Source: CAD feature listing. Evaluate the final solid. Frame: model axes, mm. Face numbers are marked on the shaded views. A direction names the side the tool comes from. Give positions to 0.01 mm unless a question says otherwise; leave off trailing zeros.
from build123d import *

# Parameters (mm, degrees)
SKETCH1_R           = 21
SKETCH1_R_2         = 12
BOSS_EXTRUDE1_DEPTH = 45
SKETCH4_RX          = 60
SKETCH4_RY          = 36
SKETCH4_R           = 6
SKETCH4_R_2         = 12
BOSS_EXTRUDE2_DEPTH = 15
SKETCH5_R           = 25
BOSS_EXTRUDE3_DEPTH = 9


with BuildPart() as part:
    # Sketch1 → Boss-Extrude1 (new body)
    with BuildSketch(Plane(origin=(0, 0, 0), x_dir=(1, 0, 0), z_dir=(0, 1, 0))):
        with Locations(Location((0, 0, 0), (0, 0, 90))):
            Circle(SKETCH1_R)
        with Locations(Location((0, 0, 0), (0, 0, 90))):
            Circle(SKETCH1_R_2, mode=Mode.SUBTRACT)
    extrude(amount=BOSS_EXTRUDE1_DEPTH)

    # Sketch4 → Boss-Extrude2 (add)
    with BuildSketch(Plane(origin=(0, 45, 0), x_dir=(1, 0, 0), z_dir=(0, 1, 0))):
        with Locations((0, 0)):
            Ellipse(SKETCH4_RX, SKETCH4_RY)
        with Locations(Location((-42, 0, 0), (0, 0, 270))):
            Circle(SKETCH4_R, mode=Mode.SUBTRACT)
        with Locations(Location((42, 0, 0), (0, 0, 90))):
            Circle(SKETCH4_R, mode=Mode.SUBTRACT)
        with Locations(Location((0, 0, 0), (0, 0, 90))):
            Circle(SKETCH4_R_2, mode=Mode.SUBTRACT)
    extrude(amount=BOSS_EXTRUDE2_DEPTH)

    # Sketch5 → Boss-Extrude3 (add)
    with BuildSketch(Plane(origin=(0, 60, 0), x_dir=(1, 0, 0), z_dir=(0, 1, 0))):
        with Locations(Location((0, 0, 0), (0, 0, 270))):
            Circle(SKETCH5_R)
    extrude(amount=BOSS_EXTRUDE3_DEPTH)

    # Sketch6 → Cut-Revolve1 (revolve, cut)
    with BuildSketch(Plane.XY, mode=Mode.PRIVATE) as cut_revolve1_sk:
        with BuildLine():
            Line((-11.5, 57.5), (0, 57.5))
            Line((0, 57.5), (0, 80.5))
            Line((0, 80.5), (-11.5, 80.5))
            ThreePointArc((-11.5, 80.5), (-23, 69), (-11.5, 57.5))
        make_face()
    revolve(cut_revolve1_sk.sketch.rotate(Axis((0, 0, 0), (0, 1, 0)), 270), axis=Axis((0, 0, 0), (0, 1, 0)), mode=Mode.SUBTRACT)

    # Sketch7 → Cut-Revolve2 (revolve, cut)
    with BuildSketch(Plane.XY, mode=Mode.PRIVATE) as cut_revolve2_sk:
        Polygon((0, 0), (-21, 0), (0, 5.626933041), align=None)
    revolve(cut_revolve2_sk.sketch.rotate(Axis((0, 0, 0), (0, 1, 0)), 270), axis=Axis((0, 0, 0), (0, 1, 0)), mode=Mode.SUBTRACT)


solid = part.part
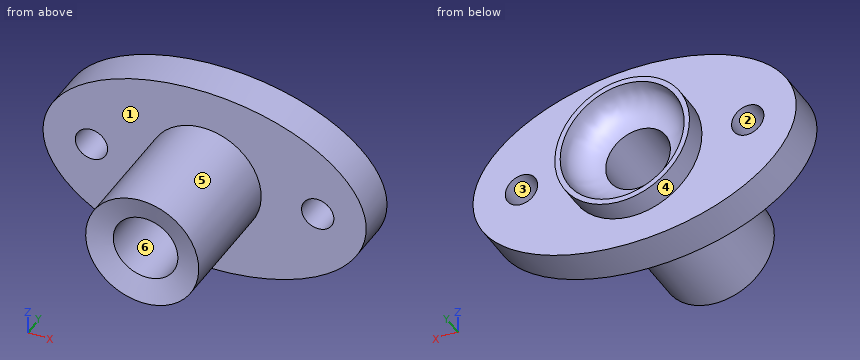
1) Reachability of the marked faces 5 and 6 from +Z, -Z, +X, -X, +Y, -Y: full face, straight path, thin tool, end or side. Return the list, or none.
Checks:
face 5: -Y
face 6: +Y, -Y
2) Ray query, probe 1 along X at (y, z) = (51.5, 0); probe 2 along X at (y, z) = (40, 0); probe 3 along Y at (x, z) = (-24.5, -1). Return the intervals inside material, ascending.
Checks:
probe 1: x = -60 to -48, -36 to -12, 12 to 36, 48 to 60
probe 2: x = -21 to -12, 12 to 21
probe 3: y = 45 to 69
3) Contact query for flat-ended pins moving along their axis: P1, Ø15.5, axis at x = -42, z = 0, coming from the +Y side; P2, Ø6, axis at x = -1.5, y = 58.5, coming from the -Z side; P3, Ø5, axis at y = 23.5, z = 3.5, coming from the -X side; P4, Ø4, axis at x = -18, y = 54, coming from the -Z side. Output: stop coordinate, or through.
Checks:
P1: stops at y = 60
P2: stops at z = -36
P3: stops at x = -20.98
P4: stops at z = -34.7
4) Pull-direction query (X, two-part tool) for the marked faces 1, 2, 3 and 4; classes: released by +X, released by -X, zero draft, split by the parting line, or undercut.
Checks:
face 1: zero draft
face 2: undercut
face 3: undercut
face 4: split by the parting line
5) Cut plane A-A (z = 0). State how many separate pieces and enclosed holes the cut face has, and give its area (3 significant figures).
Checks:
separate pieces: 4
enclosed holes: 0
area: 1,910 mm2
